Solid Edge part; units mm, degrees
sketch "Sketch1" plane through (0, 0, 0) normal (0, -1, 0) x (1, 0, 0)
  line L0 (0, 17) -> (-7.5, 17)
  line L1 (-7.5, 17) -> (-7.5, 13.5178)
  arc A0 (-8.6659, 12.8017) -> (-7.5, 13.5178) centre (0, 0) cw
  line L2 (-8.6659, 12.8017) -> (-8.6659, 10.9956)
  line L3 (8.6659, 12.8017) -> (8.6659, 10.9956)
  line L4 (7.5, 17) -> (7.5, 13.5178)
  line L5 (7.5, 17) -> (0, 17)
  arc A1 (8.6659, 10.9956) -> (-8.6659, 10.9956) centre (0, 0) cw
  arc A2 (7.5, 13.5178) -> (8.6659, 12.8017) centre (0, 0) cw
extrude "Protrusion1" add sketch "Sketch1" along normal blind 19
sketch "Sketch2" plane through (0, 0, 0) normal (0, -1, 0) x (1, 0, 0)
  line L0 (-17.5, 3.5) -> (-13.5554, 3.5)
  line L1 (-13.5554, 3.5) -> (-13.5554, -3.5)
  line L2 (-13.5554, -3.5) -> (-17.5, -3.5)
  arc A0 (-17.5, -3.5) -> (-17.5, 3.5) centre (-17.5, 0) cw
  circle A1 centre (-17.5, 0) radius 2
  line L3 (17.5, -3.5) -> (13.5554, -3.5)
  line L4 (13.5554, 3.5) -> (13.5554, -3.5)
  line L5 (13.5554, 3.5) -> (17.5, 3.5)
  arc A2 (17.5, 3.5) -> (17.5, -3.5) centre (17.5, 0) cw
  circle A3 centre (17.5, 0) radius 2
extrude "ProtrusiónExtruida_2" add sketch "Sketch2" along normal blind 1
sketch "Sketch3" plane through (0, 0, 0) normal (0, -1, 0) x (1, 0, 0)
  circle A0 centre (0, -6.5) radius 4.5
extrude "ProtrusiónExtruida_3" add sketch "Sketch3" against normal blind 2
sketch "Sketch4" plane through (0, 0, 0) normal (0, -1, 0) x (1, 0, 0)
  circle A0 centre (0, -6.5) radius 2.5
extrude "ProtrusiónExtruida_4" add sketch "Sketch4" against normal blind 9
sketch "Sketch5" plane through (0, 9, -6.5) normal (0, 1, 0) x (-1, 0, 0)
  line L0 (3.0106, 1.5) -> (-3.0106, 1.5)
  line L1 (-3.0106, 1.5) -> (-3.0106, 2.8857)
  line L2 (-3.0106, 2.8857) -> (3.0106, 2.8857)
  line L3 (3.0106, 2.8857) -> (3.0106, 1.5)
  line L4 (-3.0106, -1.5) -> (3.0106, -1.5)
  line L5 (3.0106, -1.5) -> (3.0106, -2.7741)
  line L6 (3.0106, -2.7741) -> (-3.0106, -2.7741)
  line L7 (-3.0106, -2.7741) -> (-3.0106, -1.5)
extrude "VaciadoExtruido_1" cut sketch "Sketch5" against normal blind 6
Input: part model. Units: mm. Frame: model coordinates. A direction names the side the tool comes from. Round coordinates to 2 decimals unless told otherwise and drop trailing zeros. Loops run counter-clockwise (first coordinate to the right, second up) from the corner with the lowest first, then second, coordinate; pieces in that order, holes last. Notation, with made-up numbers: (63, 83.25) -> (92, 83.25) arc R31 ccw to (92, 120.25) -> close; hole circle Ø11 at (70, -37). An arc over 180 degrees is marked (long way). Write each question's results on one line, items separated by ' | '.
1. Section A-A (z = 0). Return loops of the section in (x, y), and give its area (3 significant figures).
Geometry results:
outline: (-21, -1) -> (-19.5, -1) -> (-19.5, 0) -> (-21, 0) -> close; (-15.5, -1) -> (-14, -1) -> (-14, -19) -> (14, -19) -> (14, -1) -> (15.5, -1) -> (15.5, 0) -> (-15.5, 0) -> close; (19.5, -1) -> (21, -1) -> (21, 0) -> (19.5, 0) -> close | area: 538 mm2
2. Ray query, line 1 (Z direction, x = -17.5, y = -0.25); line 2 (Y direction, x = 6, z = 8); line 3 (Z direction, x = 2.5, y = -12.25). Return the intervals inside material, ascending. Write a range as from..to.
Geometry results:
line 1: -3.5..-2, 2..3.5 | line 2: -19..0 | line 3: -13.77..17
3. Mould query, pull axis Z, two halves, no side actions, for faces 4 (the face through (2.31, 4.67, -7.46)), 5 (the face through (0, -9, 17)), 6 (the face through (15.9, -0.5, 1.2)). Classes: +Z half, -Z half, draft (parallel to the pull), parting line (faces both ways), or undercut.
Geometry results:
face 4: parting line | face 5: +Z half | face 6: undercut
4. Set-up query: faces 1 (the face through (2.08, 0.99, -10.49)), 2 (the face through (0, -9, -14)), 3 (the face through (-15.6, -0.5, 3.5)). Return all of +Z, -Z, +X, -X, +Y, -Y with unobstructed straight access to the full face (end or side cutting, diameter ignored); none if empty.
Geometry results:
face 1: +Y | face 2: -Y | face 3: +Z, -X, +Y, -Y
5. First-contact query: P1, Ø1, axis at x = -7.5, y = -10, coming from the -Z side; P2, Ø5, axis at x = 17.5, z = 0, coming from the -Y side; P3, Ø1.5, axis at x = -11, y = -13.5, coming from the +Z side. Flat tips, straight axial feed; report the tip coordinate or a pass-through.
Geometry results:
P1: z = -12.12 | P2: y = -1 | P3: z = 9.54
6. Section C-C (y = -13.75). Return loops of the section in (x, z), and give its area (3 significant figures).
Geometry results:
outline: (-8.67, 11) arc R14 ccw (long way) to (8.67, 11) -> (8.67, 12.8) arc R15.46 ccw to (7.5, 13.52) -> (7.5, 17) -> (-7.5, 17) -> (-7.5, 13.52) arc R15.46 ccw to (-8.67, 12.8) -> close | area: 675 mm2
7. Section B-B (x = -18). Return loops of the section in (y, z), and give its area (3 significant figures).
Geometry results:
outline: (-1, -3.46) -> (0, -3.46) -> (0, -1.94) -> (-1, -1.94) -> close; (-1, 1.94) -> (0, 1.94) -> (0, 3.46) -> (-1, 3.46) -> close | area: 3.06 mm2
8. Section D-D (x = 3.5). Return loops of the section in (y, z), and give its area (3 significant figures).
Geometry results:
outline: (-19, -13.56) -> (0, -13.56) -> (0, -9.33) -> (2, -9.33) -> (2, -3.67) -> (0, -3.67) -> (0, 17) -> (-19, 17) -> close | area: 592 mm2
